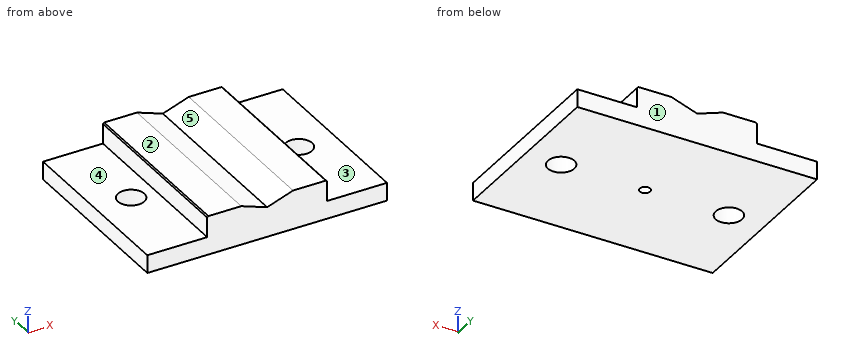
Autodesk Inventor part; units mm, degrees
ref_plane "YZ Plane" through (0, 0, 0) normal (1, 0, 0) x (0, 1, 0)
ref_plane "XZ Plane" through (0, 0, 0) normal (0, 1, 0) x (-1, 0, 0)
ref_plane "XY Plane" through (0, 0, 0) normal (0, 0, 1) x (1, 0, 0)
sketch "Sketch2" plane through (0, 0, 0) normal (0, 0, 1) x (1, 0, 0)
  line L0 (0, 0) -> (200, 0)
  line L1 (200, 0) -> (200, 150)
  line L2 (200, 150) -> (0, 150)
  line L3 (0, 150) -> (0, 0)
  dimension "d4" = 150
  dimension "d5" = 200
extrude "Extrusion2" add sketch "Sketch2" against normal blind 15
sketch "Sketch3" plane through (0, 0, 0) normal (0, 0, 1) x (1, 0, 0)
  line L0 (200, 150) -> (0, 150)
  line L1 (0, 150) -> (0, 0)
  point P0 (30, 75)
  point P1 (170, 75)
  dimension "d11" = 75
  dimension "d12" = 75
  dimension "d13" = 140
  dimension "d14" = 30
hole "Hole1" at (30, 75, 0) at (170, 75, 0) direction (0, 0, -1) diameter 22.05 end through all
sketch "Sketch6" plane through (0, 150, 0) normal (0, 1, 0) x (1, 0, 0)
  line L0 (0, 0) -> (200, 0)
  line L1 (50, 0) -> (150, 0)
  line L2 (150, 0) -> (150, -17.5)
  line L3 (50, -17.5) -> (50, 0)
  line L4 (0, 0) -> (0, 15)
  line L5 (150, -17.5) -> (121.618, -17.5)
  line L6 (121.618, -17.5) -> (100, -10)
  line L7 (100, -10) -> (78.382, -17.5)
  line L8 (78.382, -17.5) -> (50, -17.5)
  line L9 (0, 15) -> (200, 15)
  line L10 (200, 0) -> (200, 15)
  dimension "d36" = 50
  dimension "d37" = 100
  dimension "d42" = 17.5
  dimension "d45" = 28.382
  dimension "d81" = 7.5
extrude "Extrusion3" add sketch "Sketch6" against normal blind 150 contours L0 L2 L5 L6 L7 L8 L3
chamfer "Chamfer1" distance 1 angle 45 2 edges at (150, 75, 17.5) (50, 75, 17.5)
sketch "Sketch7" plane through (0, 0, -15) normal (0, 0, -1) x (-1, 0, 0)
  line L0 (-100, 150) -> (-100, 0)
  line L1 (-200, 0) -> (0, 0)
  line L2 (0, 0) -> (0, 150)
  point P0 (-100, 75)
  dimension "d54" = 75
  dimension "d55" = 100
hole "Hole3" at (100, 75, -15) direction (0, 0, 1) diameter 8.647 depth 12 tip angle 137
properties part number "Soporte Superior Tubos"
Model file for the job. Use its own axes, mm. Face numbers are marked on the shaded views. A direction names the side the tool comes from. Give positions to 0.01 mm unless a question says otherwise; leave off trailing zeros. Order: outer loops, then holes, each group sorted by start corner. A loop starts at its lowest first (then second) coordinate and runs counter-clockwise, first axis right, second up. Notation, with made-up numbers: (-19, 36) -> (11, 36) arc R31 ccw to (11, 75) -> close; hole circle Ø9 at (64.25, 10). An arc over 180 degrees is marked (long way). Use CSV: the item, a comma, the result in double quotes.
1. Band-saw the part on C-C, the plane z = 3. Give the cut face in (x, y).
Outcome:
outline,"(50, 0) -> (150, 0) -> (150, 150) -> (50, 150) -> close"
2. 3-axis set-ups, long thin cutter, end or side, ignore diameter. For the marked faces 1, 2, 3, 4 and 5: which of +Z, -Z, +X, -X, +Y, -Y reach the whole face in a straight line?
Outcome:
face 1,"+Z, -Z, +X, -X, +Y"
face 2,"+Z, +X, -X, +Y, -Y"
face 3,"+Z, +X, +Y, -Y"
face 4,"+Z, -X, +Y, -Y"
face 5,"+Z, +Y, -Y"
3. Band-saw the part on A-A, the plane x = 30. Give the cut face in (y, z) (3 decimals), then the cut area to 3 significant figures.
Outcome:
outline,"(0, -15) -> (63.975, -15) -> (63.975, 0) -> (0, 0) -> close; (86.025, -15) -> (150, -15) -> (150, 0) -> (86.025, 0) -> close"
area,"1,920 mm²"
4. Drop flat-ended pins along their axis: pin 1 (8 mm diameter, centred on y = 87, z = 12, fed in from +X); pin 2 (15 mm diameter, centred on x = 14.5, y = 79.5, fed in from +Z); pin 3 (13 mm diameter, centred on y = 103.5, z = 9.5, fed in from -X); pin 4 (1.5 mm diameter, centred on y = 39, z = 0.5, fed in from -X). Give the stop position or say it passes through.
Outcome:
pin 1,"x = 150"
pin 2,"z = 0"
pin 3,"x = 50"
pin 4,"x = 0"
5. Drill centre lines: line 1 along X through (y, z) = (75, -8.25) (1 decimal); line 2 along Y through (x, z) = (100, -10); line 3 along Y through (x, z) = (170, -4.5) (3 decimals). Where is each one in solid material? Low to high. Write a range as from..to.
Outcome:
line 1,"0..19, 41..95.7, 104.3..159, 181..200"
line 2,"0..70.68, 79.32..150"
line 3,"0..63.975, 86.025..150"
6. Band-saw the part on B-B, the plane y = 119. Give the cut face in (x, z).
Outcome:
outline,"(0, -15) -> (200, -15) -> (200, 0) -> (150, 0) -> (150, 16.5) -> (149, 17.5) -> (121.62, 17.5) -> (100, 10) -> (78.38, 17.5) -> (51, 17.5) -> (50, 16.5) -> (50, 0) -> (0, 0) -> close"
